from build123d import *

# Parameters (mm, degrees)
BOSS_EXTRUDE1_DEPTH                           = 3.175
MIRROR2_COPY_1_DEPTH                          = 3.175
INTERNAL_SHARPS_R                             = 9.525
BRAKE_MOUNT_DEPTH                             = 3.175
FILLET1_R                                     = 6.35
BEARING_POCKET_REACH                          = 100.936
SKETCH6_R                                     = 6.35
IMU_MOUNTING_DEPTH                            = 3.175
IMU_MOUNTING_HOLES_AT_2_COUNT                 = 2
IMU_MOUNTING_HOLES_AT_2_PITCH                 = 21.59
FILLET4_R                                     = 6.35
CSK_FOR_4_FLAT_HEAD_MACHINE_SCREW2_AT_2_COUNT = 2
CSK_FOR_4_FLAT_HEAD_MACHINE_SCREW2_AT_2_PITCH = 15.875
CSK_FOR_4_FLAT_HEAD_MACHINE_SCREW2_AT_3_COUNT = 2
CSK_FOR_4_FLAT_HEAD_MACHINE_SCREW2_AT_3_PITCH = 18.513272266
CSK_FOR_4_FLAT_HEAD_MACHINE_SCREW2_AT_4_COUNT = 2
CSK_FOR_4_FLAT_HEAD_MACHINE_SCREW2_AT_4_PITCH = 9.525


with BuildPart() as part:
    # Sketch1 → Boss-Extrude1 (new body)
    with BuildSketch(Plane.XY):
        with BuildLine():
            Line((9.434743879, 15.24), (0, 15.24))
            Line((0, 15.24), (0, 0))
            Line((0, 0), (12.7, 0))
            Line((12.7, 0), (12.7, 12.892596045))
            Line((12.7, 12.892596045), (51.712045103, 51.904641149))
            ThreePointArc((51.712045103, 51.904641149), (62.784313673, 54.107052302), (69.05625, 44.720436252))
            Line((69.05625, 44.720436252), (69.05625, 0))
            Line((69.05625, 0), (73.025, 0))
            Line((73.025, 0), (73.025, 57.15))
            Line((73.025, 57.15), (69.85, 57.15))
            Line((69.85, 57.15), (69.85, 60.325))
            ThreePointArc((69.85, 60.325), (65.930039796, 66.191635031), (59.009871939, 64.815128061))
            Line((59.009871939, 64.815128061), (9.434743879, 15.24))
        make_face()
    boss_extrude1 = extrude(amount=BOSS_EXTRUDE1_DEPTH)

    # Sketch11 → CSK for _4 Flat Head Machine Screw1 (revolve, cut)
    with BuildSketch(Plane(origin=(63.5, 60.325, 3.175), x_dir=(0, -1, 0), z_dir=(1, 0, 0))):
        Polygon((0, 0), (0, 3.175), (1.4732, 3.175), (1.4732, 2.030745349), (3.2385, 0), align=None)
    csk_for_4_flat_head_machine_screw1 = revolve(axis=Axis((63.5, 60.325, 9.525), (0, 0, -1)), mode=Mode.SUBTRACT)

    # Mirror1: Boss-Extrude1, CSK for _4 Flat Head Machine Screw1 across plane
    add(boss_extrude1.mirror(Plane.ZX))
    add(csk_for_4_flat_head_machine_screw1.mirror(Plane.ZX), mode=Mode.SUBTRACT)

    # Mirror2: Boss-Extrude1, CSK for _4 Flat Head Machine Screw1 across plane
    add(boss_extrude1.mirror(Plane(origin=(0, 0, 0), x_dir=(0, 0, 1), z_dir=(1, 0, 0))))
    add(csk_for_4_flat_head_machine_screw1.mirror(Plane(origin=(0, 0, 0), x_dir=(0, 0, 1), z_dir=(1, 0, 0))), mode=Mode.SUBTRACT)

    # Mirror2 copy 1 sketch → Mirror2 copy 1 (add)
    with BuildSketch(Plane(origin=(0, 0, 0), x_dir=(-1, 0, 0), z_dir=(0, 0, 1))):
        with BuildLine():
            Line((9.434743879, 15.24), (0, 15.24))
            Line((0, 15.24), (0, 0))
            Line((0, 0), (12.7, 0))
            Line((12.7, 0), (12.7, 12.892596045))
            Line((12.7, 12.892596045), (51.712045103, 51.904641149))
            ThreePointArc((51.712045103, 51.904641149), (62.784313673, 54.107052302), (69.05625, 44.720436252))
            Line((69.05625, 44.720436252), (69.05625, 0))
            Line((69.05625, 0), (73.025, 0))
            Line((73.025, 0), (73.025, 57.15))
            Line((73.025, 57.15), (69.85, 57.15))
            Line((69.85, 57.15), (69.85, 60.325))
            ThreePointArc((69.85, 60.325), (65.930039796, 66.191635031), (59.009871939, 64.815128061))
            Line((59.009871939, 64.815128061), (9.434743879, 15.24))
        make_face()
    extrude(amount=MIRROR2_COPY_1_DEPTH)

    # Mirror2 copy 2 sketch → Mirror2 copy 2 (revolve, cut)
    with BuildSketch(Plane(origin=(-63.5, -60.325, 3.175), x_dir=(0, 1, 0), z_dir=(-1, 0, 0))):
        Polygon((0, 0), (0, 3.175), (1.4732, 3.175), (1.4732, 2.030745349), (3.2385, 0), align=None)
    revolve(axis=Axis((-63.5, -60.325, 9.525), (0, 0, -1)), mode=Mode.SUBTRACT)

    # INTERNAL-SHARPS
    internal_sharps_edges = [part.edges().sort_by_distance(p)[0] for p in [
        (-9.434743879, 15.24, 1.5875),
        (-12.7, 12.892596045, 1.5875),
        (9.434743879, 15.24, 1.5875),
        (12.7, 12.892596045, 1.5875),
        (9.434743879, -15.24, 1.5875),
        (12.7, -12.892596045, 1.5875),
        (-12.7, -12.892596045, 1.5875),
        (-9.434743879, -15.24, 1.5875),
    ]]
    fillet(internal_sharps_edges, radius=INTERNAL_SHARPS_R)

    # Sketch5 → BRAKE-MOUNT (add)
    with BuildSketch(Plane.XY):
        Polygon((69.05625, 12.7), (57.785, 12.7), (35.146201977, 35.338798023), (32.901137947, 33.093733992), (53.975, 12.019871939), (53.975, -12.019871939), (32.901137947, -33.093733992), (35.146201977, -35.338798023), (57.785, -12.7), (69.05625, -12.7), align=None)
    extrude(amount=BRAKE_MOUNT_DEPTH)

    # Fillet1
    fillet1_edges = [part.edges().sort_by_distance(p)[0] for p in [
        (57.785, -12.7, 1.5875),
        (69.05625, -12.7, 1.5875),
        (69.05625, 12.7, 1.5875),
        (57.785, 12.7, 1.5875),
        (35.146201977, 35.338798023, 1.5875),
        (32.901137947, 33.093733992, 1.5875),
        (53.975, 12.019871939, 1.5875),
        (53.975, -12.019871939, 1.5875),
        (32.901137947, -33.093733992, 1.5875),
        (35.146201977, -35.338798023, 1.5875),
    ]]
    fillet(fillet1_edges, radius=FILLET1_R)

    # Sketch6 → BEARING-POCKET (cut, up to next)
    with BuildSketch(Plane(origin=(0, 0, 0), x_dir=(-1, 0, 0), z_dir=(0, 0, -1)), mode=Mode.PRIVATE) as bearing_pocket_sk1:
        Circle(SKETCH6_R)
    bearing_pocket_tool1 = extrude(bearing_pocket_sk1.sketch, amount=-BEARING_POCKET_REACH, mode=Mode.PRIVATE) & part.part
    add(bearing_pocket_tool1.solids().sort_by_distance((0, 0, 0))[0], mode=Mode.SUBTRACT)

    # Sketch13 → IMU-MOUNTING (add)
    with BuildSketch(Plane.XY):
        with BuildLine():
            Line((-73.025, 44.45), (-73.025, 12.7))
            Line((-73.025, 12.7), (-67.945, 12.7))
            ThreePointArc((-67.945, 12.7), (-62.895851895, 18.339020045), (-69.05625, 22.736967161))
            Line((-69.05625, 22.736967161), (-69.05625, 34.413032839))
            ThreePointArc((-69.05625, 34.413032839), (-62.895851895, 38.810979955), (-67.945, 44.45))
            Line((-67.945, 44.45), (-73.025, 44.45))
        make_face()
    extrude(amount=IMU_MOUNTING_DEPTH)

    # Sketch15 → IMU-MOUNTING-HOLES (revolve, cut)
    with BuildSketch(Plane(origin=(-67.945, 17.78, 3.175), x_dir=(0, -1, 0), z_dir=(1, 0, 0))):
        Polygon((0, 0), (0, 3.175), (1.4732, 3.175), (1.4732, 2.030745349), (3.2385, 0), align=None)
    imu_mounting_holes = revolve(axis=Axis((-67.945, 17.78, 9.525), (0, 0, -1)), mode=Mode.SUBTRACT)

    # IMU-MOUNTING-HOLES at 2: IMU-MOUNTING-HOLES ×2
    with Locations(*[(0, i * IMU_MOUNTING_HOLES_AT_2_PITCH, 0) for i in range(1, IMU_MOUNTING_HOLES_AT_2_COUNT)]):
        add(imu_mounting_holes, mode=Mode.SUBTRACT)

    # Fillet4
    # the kernel refuses this fillet: 6.35 mm, written as the material it adds along each edge
    with BuildSketch(Plane(origin=(-69.05625, 12.7, 0), x_dir=(0, -1, 0), z_dir=(0, 0, 1))) as fillet4_piece_1:
        with BuildLine():
            CenterArc((5.07875969, 6.35), FILLET4_R, 207.279612736, 62.720387264)
            Line((-0.564995693, 3.439583333), (-1.129371232, 3.148541667))
            ThreePointArc((-1.129371232, 3.148541667), (-0.635, 1.11125), (-0.635, 0))
            Line((-0.635, 0), (0, -0.635))
            Line((0, -0.635), (5.07875969, -0.635))
            Line((5.07875969, -0.635), (5.07875969, 0))
        make_face()
    extrude(amount=3.175)
    with BuildSketch(Plane(origin=(-69.05625, 44.45, 3.175), x_dir=(0.9650860759798715, -0.26193294170411996, 0), z_dir=(0, 0, -1))) as fillet4_piece_2:
        with BuildLine():
            CenterArc((7.197142212, -5.764455356), FILLET4_R, 114.798529297, 113.445685193)
            Line((2.968315283, -10.501492701), (2.54543259, -10.975196435))
            ThreePointArc((2.54543259, -10.975196435), (-0.683665821, -0.094666843), (-0.612829658, 0.166327418))
            Line((-0.612829658, 0.166327418), (0.166327418, 0.612829658))
            ThreePointArc((0.166327418, 0.612829658), (1.23877932, 0.321756677), (4.267432177, 0.576445536))
            Line((4.267432177, 0.576445536), (4.533769453, 0))
        make_face()
    extrude(amount=3.175)
    with BuildSketch(Plane(origin=(-69.05625, 22.736967161, 0), x_dir=(0.9918455939072564, -0.12744535239372892, 0), z_dir=(0, 0, 1))) as fillet4_piece_3:
        with BuildLine():
            CenterArc((5.635275239, 5.968652988), FILLET4_R, 187.321993821, 62.720387264)
            Line((-0.662944282, 5.159375), (0, 0))
            ThreePointArc((0, 0), (1.733930843, 0.30507761), (3.467861686, 0))
        make_face()
    extrude(amount=3.175)
    with BuildSketch(Plane(origin=(-69.05625, 34.413032839, 0), x_dir=(0, -1, 0), z_dir=(0, 0, 1))) as fillet4_piece_4:
        with BuildLine():
            CenterArc((5.201792529, 6.35), FILLET4_R, 207.279612736, 62.720387264)
            ThreePointArc((-0.441962855, 3.439583333), (0.081608456, 1.75867239), (0, 0))
            Line((0, 0), (5.201792529, 0))
        make_face()
    extrude(amount=3.175)

    # Sketch17 → CSK for _4 Flat Head Machine Screw2 (revolve, cut)
    with BuildSketch(Plane(origin=(58.7375, -7.9375, 3.175), x_dir=(0, -1, 0), z_dir=(1, 0, 0))):
        Polygon((0, 0), (0, 3.175), (1.4732, 3.175), (1.4732, 2.030745349), (3.2385, 0), align=None)
    csk_for_4_flat_head_machine_screw2 = revolve(axis=Axis((58.7375, -7.9375, 9.525), (0, 0, -1)), mode=Mode.SUBTRACT)

    # CSK for _4 Flat Head Machine Screw2 at 2: CSK for _4 Flat Head Machine Screw2 ×2
    with Locations(*[(0, i * CSK_FOR_4_FLAT_HEAD_MACHINE_SCREW2_AT_2_PITCH, 0) for i in range(1, CSK_FOR_4_FLAT_HEAD_MACHINE_SCREW2_AT_2_COUNT)]):
        add(csk_for_4_flat_head_machine_screw2, mode=Mode.SUBTRACT)

    # CSK for _4 Flat Head Machine Screw2 at 3: CSK for _4 Flat Head Machine Screw2 ×2
    with Locations(*[Vector(0.5144957554275265, 0.8574929257125442, 0) * (i * CSK_FOR_4_FLAT_HEAD_MACHINE_SCREW2_AT_3_PITCH) for i in range(1, CSK_FOR_4_FLAT_HEAD_MACHINE_SCREW2_AT_3_COUNT)]):
        add(csk_for_4_flat_head_machine_screw2, mode=Mode.SUBTRACT)

    # CSK for _4 Flat Head Machine Screw2 at 4: CSK for _4 Flat Head Machine Screw2 ×2
    with Locations(*[(i * CSK_FOR_4_FLAT_HEAD_MACHINE_SCREW2_AT_4_PITCH, 0, 0) for i in range(1, CSK_FOR_4_FLAT_HEAD_MACHINE_SCREW2_AT_4_COUNT)]):
        add(csk_for_4_flat_head_machine_screw2, mode=Mode.SUBTRACT)


solid = part.part
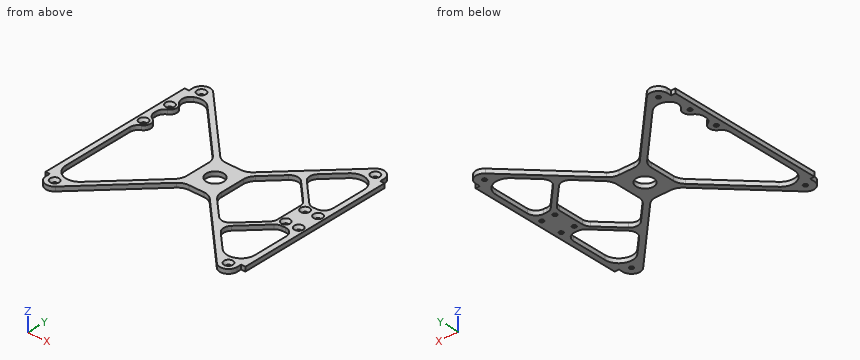
Design review of the part built by this model. Coordinates are the model's own, in mm. Round coordinates to 2 decimals unless told otherwise and drop trailing zeros. Loops run counter-clockwise (first coordinate to the right, second up) from the corner with the lowest first, then second, coordinate; pieces in that order, holes last. Notation, with made-up numbers: (-40, -26) -> (13, -26) arc R22 cw to (13, 5) -> close; hole circle Ø7 at (-33, -21). An arc over 180 degrees is marked (long way). Use one line per item in the form item = value. Start each with the question number.
Q1. We need section A-A on x = 0. Give the boundary of the cut face in (y, z) (3 decimals), then the cut area to 3 significant figures.
Q2. We need section D-D on x = -20. Give the boundary of the cut face in (y, z) (3 decimals), then the cut area to 3 significant figures.
Q3. We need section B-B on y = 0. Give the boundary of the cut face in (x, z) (3 decimals), then the cut area to 3 significant figures.
Q4. For pin 1 Ø20.5 at (x, y) = (0, 0) entering from +Z (3 decimals); pin 2 Ø1.8 at (x, y) = (58.74, -7.94) entering from -Z; pin 3 Ø1.8 at (x, z) = (62, 1) entering from -Y, all flat-tipped, find the tip position at first contact; note any pin that passes through.
Q5. We need section C-C on x = 46.5. Give the boundary of the cut face in (y, z) (3 decimals).
Q6. Wall thickness on line 1 along X through (y, z) = (11, 0.5) (3 decimals); line 2 along X through (y, z) = (38.5, 1.05) (3 decimals); line 3 along X through (y, z) = (-19.5, 1.25) (3 decimals): over which ranges is each line inside the solid? List them lowest first. Write a range as [from, to].
Calculated:
q1.outline = (-15.24, 0) -> (-6.35, 0) -> (-6.35, 3.175) -> (-15.24, 3.175) -> close; (6.35, 0) -> (15.24, 0) -> (15.24, 3.175) -> (6.35, 3.175) -> close
q1.area = 56.5 mm²
q2.outline = (-25.805, 0) -> (-20.193, 0) -> (-20.193, 3.175) -> (-25.805, 3.175) -> close; (20.193, 0) -> (25.805, 0) -> (25.805, 3.175) -> (20.193, 3.175) -> close
q2.area = 35.6 mm²
q3.outline = (-73.025, 0) -> (-69.056, 0) -> (-69.056, 3.175) -> (-73.025, 3.175) -> close; (-12.7, 0) -> (-6.35, 0) -> (-6.35, 3.175) -> (-12.7, 3.175) -> close; (6.35, 0) -> (12.7, 0) -> (12.7, 3.175) -> (6.35, 3.175) -> close; (53.975, 0) -> (73.025, 0) -> (73.025, 3.175) -> (53.975, 3.175) -> close
q3.area = 113 mm²
q4.pin_1 = 3.175
q4.pin_2 = through
q4.pin_3 = -66.65
q5.outline = (-52.305, 0) -> (-46.693, 0) -> (-46.693, 3.175) -> (-52.305, 3.175) -> close; (-23.985, 0) -> (-19.495, 0) -> (-19.495, 3.175) -> (-23.985, 3.175) -> close; (19.495, 0) -> (23.985, 0) -> (23.985, 3.175) -> (19.495, 3.175) -> close; (46.693, 0) -> (52.305, 0) -> (52.305, 3.175) -> (46.693, 3.175) -> close
q6.line_1 = [-73.025, -68.083], [-12.924, 12.924], [53.767, 73.025]
q6.line_2 = [-73.025, -69.134], [-66.756, -62.94], [-38.307, -32.695], [32.695, 38.619], [69.056, 73.025]
q6.line_3 = [-73.025, -69.056], [-19.307, -13.695], [13.695, 19.307], [46.495, 50.985], [69.056, 73.025]
